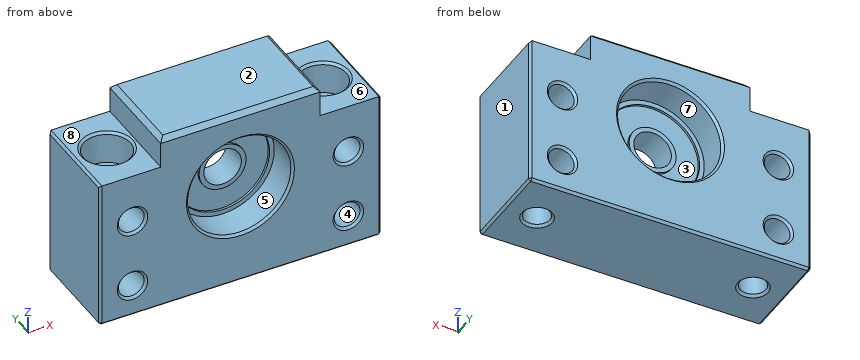
```python
from build123d import *

# Parameters (mm, degrees)
SKETCH_R         = 11
PAD_DEPTH        = 10
SKETCH001_R      = 2.75
POCKET_DEPTH     = 20.001
SKETCH003_R      = 5
POCKET001_DEPTH  = 7
SKETCH004_R      = 2.75
POCKET002_DEPTH  = 39.001
CHAMFER_SIZE     = 1
CHAMFER001_SIZE  = 0.5
CHAMFER002_SIZE  = 0.5
CHAMFER003_SIZE  = 0.5
CHAMFER004_SIZE  = 0.5
CHAMFER005_SIZE  = 0.5
REVOLUTION_ANGLE = 360


with BuildPart() as housing_h_holes_chamfer:
    # Sketch → Pad (new body, symmetric)
    with BuildSketch(Plane.XZ):
        Polygon((-30, 32.5), (-30, 0), (30, 0), (30, 32.5), (17, 32.5), (17, 39), (-17, 39), (-17, 32.5), align=None)
        with Locations((0, 22)):
            Circle(SKETCH_R, mode=Mode.SUBTRACT)
    extrude(amount=PAD_DEPTH, both=True)

    # Sketch001 → Pocket (cut, through all)
    with BuildSketch(Plane.XZ.offset(10)):
        with Locations((-23, 22)):
            Circle(SKETCH001_R)
        with Locations((23, 22)):
            Circle(SKETCH001_R)
        with Locations((-23, 7)):
            Circle(SKETCH001_R)
        with Locations((23, 7)):
            Circle(SKETCH001_R)
    extrude(amount=-POCKET_DEPTH, mode=Mode.SUBTRACT)

    # Sketch003 → Pocket001 (cut)
    with BuildSketch(Plane(origin=(0, 0, 32.5), x_dir=(-1, 0, 0), z_dir=(0, 0, 1))):
        with Locations((-23, 0)):
            Circle(SKETCH003_R)
        with Locations((23, 0)):
            Circle(SKETCH003_R)
    extrude(amount=-POCKET001_DEPTH, mode=Mode.SUBTRACT)

    # Sketch004 → Pocket002 (cut, through all)
    with BuildSketch(Plane(origin=(0, 0, 0), x_dir=(1, 0, 0), z_dir=(0, 0, -1))):
        with Locations((-23, 0)):
            Circle(SKETCH004_R)
        with Locations((23, 0)):
            Circle(SKETCH004_R)
    extrude(amount=-POCKET002_DEPTH, mode=Mode.SUBTRACT)

    # Chamfer
    chamfer_edges = [housing_h_holes_chamfer.edges().sort_by_distance(p)[0] for p in [
        (-17, 0, 39),
        (0, 10, 39),
        (0, -10, 39),
        (17, 0, 39),
    ]]
    chamfer(chamfer_edges, length=CHAMFER_SIZE)

    # Chamfer001
    chamfer001_edges = [housing_h_holes_chamfer.edges().sort_by_distance(p)[0] for p in [
        (30, 0, 32.5),
        (30, -10, 16.25),
        (30, 10, 16.25),
        (30, 0, 0),
        (0, -10, 0),
        (0, 10, 0),
        (-30, 0, 0),
        (-30, 10, 16.25),
        (-30, 0, 32.5),
        (-30, -10, 16.25),
    ]]
    chamfer(chamfer001_edges, length=CHAMFER001_SIZE)

    # Chamfer002
    chamfer002_edges = [housing_h_holes_chamfer.edges().sort_by_distance(p)[0] for p in [
        (-11, -10, 22),
        (-11, 10, 22),
    ]]
    chamfer(chamfer002_edges, length=CHAMFER002_SIZE)

    # Chamfer003
    chamfer003_edges = [housing_h_holes_chamfer.edges().sort_by_distance(p)[0] for p in [
        (-18, 0, 32.5),
        (28, 0, 32.5),
    ]]
    chamfer(chamfer003_edges, length=CHAMFER003_SIZE)

    # Chamfer004
    chamfer004_edges = [housing_h_holes_chamfer.edges().sort_by_distance(p)[0] for p in [
        (20.25, 0, 0),
        (-25.75, 0, 0),
    ]]
    chamfer(chamfer004_edges, length=CHAMFER004_SIZE)

    # Chamfer005
    chamfer005_edges = [housing_h_holes_chamfer.edges().sort_by_distance(p)[0] for p in [
        (-25.75, -10, 22),
        (20.25, -10, 22),
        (20.25, -10, 7),
        (-25.75, -10, 7),
        (20.25, 10, 22),
        (-25.75, 10, 22),
        (-25.75, 10, 7),
        (20.25, 10, 7),
    ]]
    chamfer(chamfer005_edges, length=CHAMFER005_SIZE)


with BuildPart() as obj1:
    # Sketch002 → Revolution (revolve, symmetric)
    with BuildSketch(Plane.YZ) as revolution_sk:
        Polygon((3, 26), (-3, 26), (-3, 27), (-2.5, 27), (-2.5, 32), (-3, 32), (-3, 33), (3, 33), (3, 32), (2.5, 32), (2.5, 27), (3, 27), align=None)
    revolve(axis=Axis((0, -10, 22), (0, 1, 0)), revolution_arc=REVOLUTION_ANGLE / 2)
    revolve(revolution_sk.sketch, axis=Axis((0, -10, 22), (0, -1, 0)), revolution_arc=REVOLUTION_ANGLE / 2)

    # Fusion: union housing-h-holes-chamfer
    add(housing_h_holes_chamfer.part)


solid = obj1.part
```
Input: part model. Units: mm. Frame: model coordinates. Face numbers are marked on the shaded views. A direction names the side the tool comes from. Round coordinates to 2 decimals unless told otherwise and drop trailing zeros. Write each question's results on one line, items separated by ' | '.
Q1. Section query A-A (x = -23). State how many separate pieces and enclosed holes the cut face has, and give its area (4 significant figures).
Results:
separate pieces: 6 | enclosed holes: 0 | area: 278.5 mm^2
Q2. Line query: line 1 along Z through (x, y) = (23, -3.75); line 2 along X through (y, z) = (-6.5, 7); line 3 along Z through (x, y) = (23, 5.75). Output: solid intervals per line, ascending.
Results:
line 1: z = 0 to 4.25, 9.75 to 19.25, 24.75 to 25.5 | line 2: x = -30 to -25.75, -20.25 to 20.25, 25.75 to 30 | line 3: z = 0 to 4.25, 9.75 to 19.25, 24.75 to 32.5
Q3. Access query for the marked faces 5, 6, 7 and 8. Directions: +Z, -Z, +X, -X, +Y, -Y. A direction counts if a zero-diameter tool reaches every point of the face in a straight line with its end or side. Return the directions, or none.
Results:
face 5: -Y | face 6: +Z, +X, +Y, -Y | face 7: +Y | face 8: +Z, -X, +Y, -Y
Q4. Draft query along Z for the marked faces 1, 2, 3 and 4. Return one class per face: released by +Z, released by -Z, zero draft, split by the parting line, or undercut.
Results:
face 1: zero draft | face 2: released by +Z | face 3: undercut | face 4: undercut
Q5. Pin query (flat end, axial travel): P1, Ø11, axis at x = -24.5, y = 1.5, coming from the +Z side; P2, Ø1.5, axis at x = -22.5, z = 9, coming from the -Y side; P3, Ø11, axis at x = 4.5, z = 22, coming from the -Y side; P4, Ø5, axis at x = 23, y = 0, coming from the -Z side. Return the tip coordinate at first contact, or that it passes through.
Results:
P1: stops at z = 32.5 | P2: stops at y = -9.56 | P3: stops at y = -3 | P4: passes through
